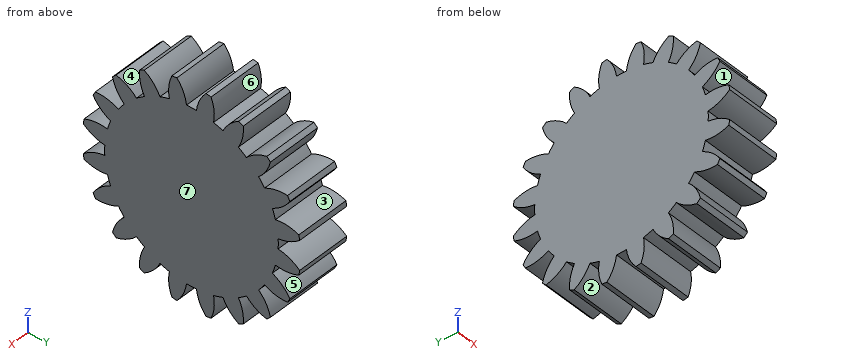
from build123d import *

# Parameters (mm, degrees)
BASPROSKE_W     = 5.5
BASPROSKE_H     = 11
TOOTHCUT_DEPTH  = 17.5
TEETHCUTS_COUNT = 20
TEETHCUTS_ANGLE = 342
BORSKE_R        = 3
BORE_DEPTH      = 50.0000508
EXTRUDE_START   = -5.5
SKETCH_1_R      = 3
EXTRUDE_1_DEPTH = 5.5


with BuildPart() as part:
    # BasProSke → Base-Revolve (revolve)
    with BuildSketch(Plane(origin=(0, 0, 0), x_dir=(1, 0, 0), z_dir=(0, 1, 0)), mode=Mode.PRIVATE) as base_revolve_sk:
        with Locations((2.75, 5.5)):
            Rectangle(BASPROSKE_W, BASPROSKE_H)
    revolve(base_revolve_sk.sketch.rotate(Axis((-10, 0, 0), (1, 0, 0)), 180), axis=Axis((-10, 0, 0), (1, 0, 0)))

    # TooCutSke → ToothCut (cut, through all)
    with BuildSketch(Plane(origin=(0, 0, 0), x_dir=(0, 0, -1), z_dir=(1, 0, 0))):
        with BuildLine():
            ThreePointArc((0.499924007, 8.734705318), (0, 8.749), (-0.499924007, 8.734705318))
            ThreePointArc((-0.499924007, 8.734705318), (-0.824302243, 9.905497836), (-1.485192705, 10.924909509))
            ThreePointArc((-1.485192705, 10.924909509), (0, 11.0254), (1.485192705, 10.924909509))
            ThreePointArc((1.485192705, 10.924909509), (0.824302243, 9.905497836), (0.499924007, 8.734705318))
        make_face()
    toothcut = extrude(amount=TOOTHCUT_DEPTH, mode=Mode.SUBTRACT)

    # TeethCuts: ToothCut ×20 about axis
    teethcuts_axis = Axis((-10, 0, 0), (1, 0, 0))
    for i in range(1, TEETHCUTS_COUNT):
        add(toothcut.rotate(teethcuts_axis, i * TEETHCUTS_ANGLE / (TEETHCUTS_COUNT - 1)), mode=Mode.SUBTRACT)

    # BorSke → Bore (cut, symmetric)
    with BuildSketch(Plane(origin=(0, 0, 0), x_dir=(0, 0, -1), z_dir=(1, 0, 0))):
        with Locations(Location((0, 0, 0), (0, 0, 180))):
            Circle(BORSKE_R)
    extrude(amount=BORE_DEPTH, both=True, mode=Mode.SUBTRACT)

    # ｽｹｯﾁ1 → ﾎﾞｽ - 押し出し1 (add)
    with BuildSketch(Plane.ZY.offset(EXTRUDE_START)):
        Circle(SKETCH_1_R)
    extrude(amount=EXTRUDE_1_DEPTH)


solid = part.part
Geometry: final body of the model. Coordinates: model frame, mm. Face numbers are marked on the shaded views. A direction names the side the tool comes from. Coordinates: 2 decimals unless noted, no trailing zeros. Loops run counter-clockwise (first coordinate to the right, second up) from the corner with the lowest first, then second, coordinate; pieces in that order, holes last. Notation, with made-up numbers: (-10.5, 14) - (13.5, 14) arc R20 ccw to (13.5, 42) - close; hole circle Ø4 at (48.25, 89). An arc over 180 degrees is marked (long way). One line per question, with ' | ' between items. Start each with the question number.
(1) Cut plane C-C on y = -4. Output: boundary loops of the cut face in (x, z).
(2) Ray query, L1, parallel to Z at x = 1.7, y = -7; L2, parallel to Z at x = 2.05, y = 7.5; L3, parallel to Z at x = 4.15, y = -9.5. Return the intervals inside material, ascending. Write a range as from..to.
(3) Cut plane A-A on z = 9. Output: boundary loops of the cut face in (x, y), and give its area (3 significant figures).
(4) First-contact query: pin 1 (3 mm diameter, centred on x = 1.5, z = -4, fed in from -Y); pin 2 (1 mm diameter, centred on x = 3, z = -6.5, fed in from -Y); pin 3 (2 mm diameter, centred on x = 4, y = -6.5, fed in from -Z). Flat tips, straight axial feed; report the tip coordinate or a pass-through.
(5) Cut plane B-B on z = -9.25. Output: boundary loops of the cut face in (x, y).
(6) Reachability of the marked faces 1, 2, 3 and 4 from +Z, -Z, +X, -X, +Y, -Y: full face, straight path, thin tool, end or side. Return the list, or none.
(7) Draft query along Y for the marked faces 5, 6 and 7. Return one class per face: +Y half, -Y half, draft (parallel to the pull), parting line (faces both ways), or undercut.
Here are the results:
1) outline: (0, -9.33) - (5.5, -9.33) - (5.5, 9.33) - (0, 9.33) - close
2) L1: -7.78..-5.77, -5.25..5.25, 5.77..7.78 | L2: -7.94..-6.44, -4.8..4.8, 6.44..7.94 | L3: -5.24..-4.19, -2.29..-0.67, 0.67..2.29, 4.19..5.24
3) outline: (0, -5.23) - (5.5, -5.23) - (5.5, -3.7) - (0, -3.7) - close; (0, -2.29) - (5.5, -2.29) - (5.5, -0.54) - (0, -0.54) - close; (0, 0.54) - (5.5, 0.54) - (5.5, 2.29) - (0, 2.29) - close; (0, 3.7) - (5.5, 3.7) - (5.5, 5.23) - (0, 5.23) - close | area: 36.1 mm²
4) pin 1: y = -9.92 | pin 2: y = -7.78 | pin 3: z = -7.94
5) outline: (0, -5.24) - (5.5, -5.24) - (5.5, -3.92) - (0, -3.92) - close; (0, -2.3) - (5.5, -2.3) - (5.5, -0.6) - (0, -0.6) - close; (0, 0.6) - (5.5, 0.6) - (5.5, 2.3) - (0, 2.3) - close; (0, 3.92) - (5.5, 3.92) - (5.5, 5.24) - (0, 5.24) - close
6) face 1: +X, -X, -Y | face 2: -Z, +X, -X | face 3: +X, -X | face 4: +Z, +X, -X
7) face 5: +Y half | face 6: undercut | face 7: draft
